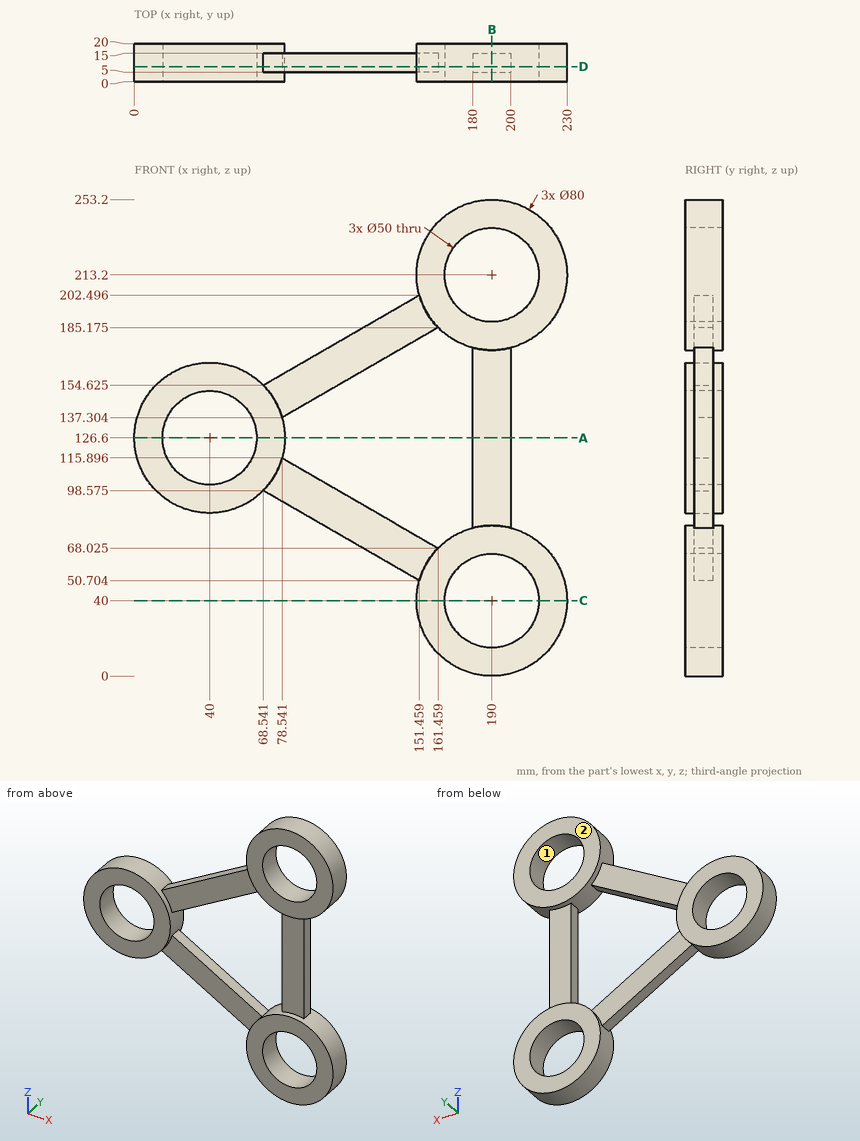
Design review of the part shown in the three views and the two pictorial views. Dimensions are in mm from the part's minimum x, y and z. Give positions to 0.01 mm unless a question says otherwise; leave off trailing zeros. Loops run counter-clockwise (first coordinate to the right, second up) from the corner with the lowest first, then second, coordinate; pieces in that order, holes last. Notation, with made-up numbers: (73, 53) -> (81, 53) arc R27 cw to (81, 89) -> close; hole circle Ø11 at (81.25, -39). An arc over 180 degrees is marked (long way). One line per item, written item: value.
Q1. Draft analysis for pull direction X (two halves, no side actions). For the marked faces 1 and 2, state which applies: pulls with the +X half, pulls with the -X half, needs draft (parallel to the pull), parting line crosses it, or undercut.
Numbers:
face 1: undercut
face 2: needs draft
Q2. We need section D-D on y = 8. Give the boundary of the cut face in (x, z) (1 decimal).
Numbers:
outline: (68.5, 98.6) -> (151.5, 50.7) arc R40 ccw (long way) to (200, 78.7) -> (200, 174.5) arc R40 ccw (long way) to (151.5, 202.5) -> (68.5, 154.6) arc R40 ccw (long way) to start; hole circle Ø50 at (40, 126.6); hole (78.5, 115.9) -> (161.5, 68) arc R40 cw to (180, 78.7) -> (180, 174.5) arc R40 cw to (161.5, 185.2) -> (78.5, 137.3) arc R40 cw to start; hole circle Ø50 at (190, 40); hole circle Ø50 at (190, 213.2)
Q3. We need section C-C on z = 40. Give the boundary of the cut face in (x, y), and give its area (3 significant figures).
Numbers:
outline: (150, 0) -> (165, 0) -> (165, 20) -> (150, 20) -> close; (215, 0) -> (230, 0) -> (230, 20) -> (215, 20) -> close
area: 600 mm^2
Q4. For pin 1 Ø6 at (x, z) = (188, 145) entering from +Y; pin 2 Ø19.5 at (x, z) = (128.5, 160.5) entering from -Y; pin 3 Ø12 at (x, y) = (175.5, 2) entering from -Z, all flat-tipped, find the tip position at first contact; note any pin that passes through.
Numbers:
pin 1: stops at y = 15
pin 2: stops at y = 5
pin 3: stops at z = 0.91
Q5. We need section B-B on x = 190. Give the boundary of the cut face in (y, z), and give its area (3 significant figures).
Numbers:
outline: (0, 0) -> (20, 0) -> (20, 15) -> (0, 15) -> close; (0, 65) -> (20, 65) -> (20, 80) -> (15, 80) -> (15, 173.2) -> (20, 173.2) -> (20, 188.2) -> (0, 188.2) -> (0, 173.2) -> (5, 173.2) -> (5, 80) -> (0, 80) -> close; (0, 238.2) -> (20, 238.2) -> (20, 253.2) -> (0, 253.2) -> close
area: 2,130 mm^2
Q6. We need section A-A on z = 126.6. Give the boundary of the cut face in (x, y).
Numbers:
outline: (0, 0) -> (15, 0) -> (15, 20) -> (0, 20) -> close; (65, 0) -> (80, 0) -> (80, 20) -> (65, 20) -> close; (180, 5) -> (200, 5) -> (200, 15) -> (180, 15) -> close
Q7. For L1, parallel to X at y = 6.75, z = 126.6; L2, parallel to X at y = 15.75, z = 126.6; L3, parallel to X at y = 10, z = 213.2, list the stretches that pass through material, from the lowest coordinate up.
Numbers:
L1: x = 0 to 15, 65 to 80, 180 to 200
L2: x = 0 to 15, 65 to 80
L3: x = 150 to 165, 215 to 230
